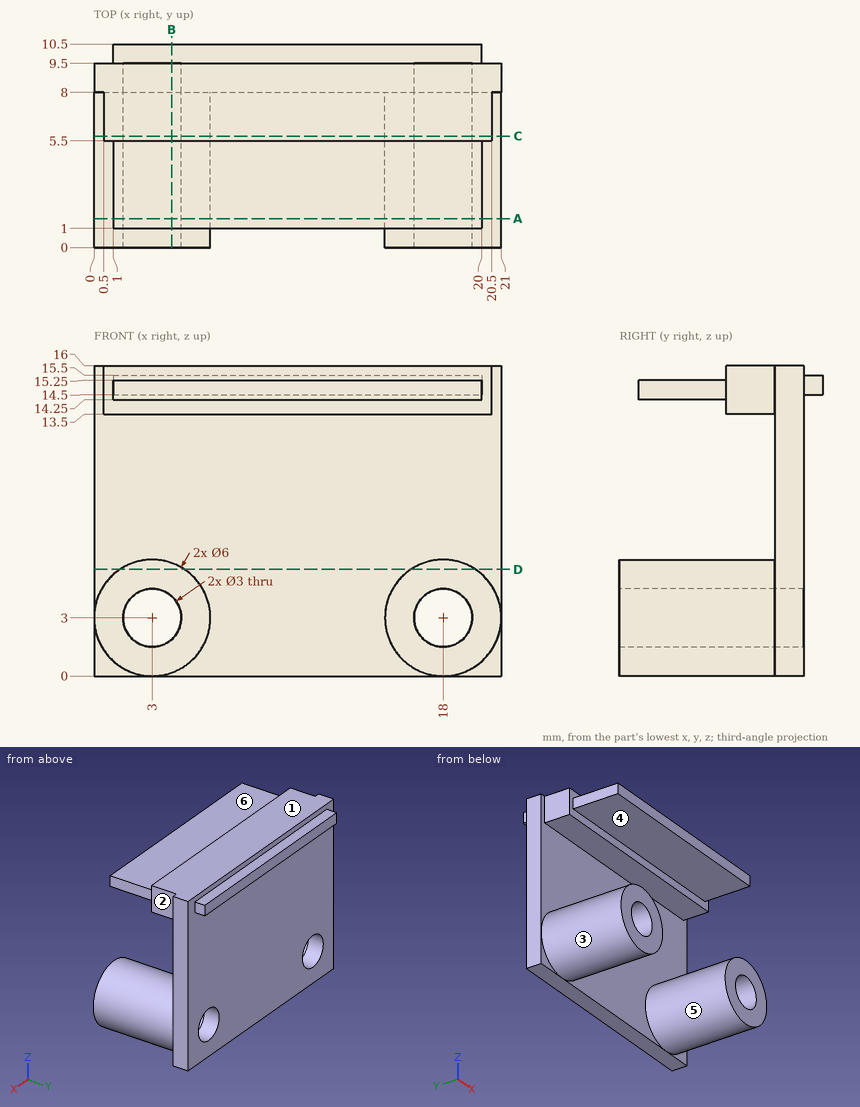
Here's the drawing with two shaded views (mm, measured from the low corner). I have some questions. A direction names the side the tool comes from. Coordinates: 2 decimals unless noted, no trailing zeros. Order: outer loops, then holes, each group sorted by start corner. A loop starts at its lowest first (then second) coordinate and runs counter-clockwise, first axis right, second up. Notation, with made-up numbers: (-13.5, 28.5) - (7.5, 28.5) arc R35 ccw to (7.5, 63.5) - close; hole circle Ø1 at (-23, 71). An arc over 180 degrees is marked (long way). Answer in a Markdown table with one row per item. Add a question column.
(1) If we section it at A-A, the plane y = 1.5: Please give me the cut outline in (x, z).
(2) If we mould it in two halves opening along Z, with no side actions, what happens to the marked faces 1, 2 and 3? For each: released by +Z, released by -Z, zero draft, split by the parting line, or undercut.
(3) I need wall thicknesses on L1, parallel to Z at x = 18, y = 6.5; L2, parallel to X at y = 2, z = 3; L3, parallel to Z at x = 2.25, y = 4.25. Which ranges of each line are inside material? Lowest first, please.
(4) Will these pins go through, and if not, where does the flat tip stop? pin 1 (0.8 mm diameter, centred on y = 7.5, z = 14.5, fed in from -X); pin 2 (1 mm diameter, centred on x = 14.5, z = 8, fed in from +Y); pin 3 (0.5 mm diameter, centred on y = 4, z = 14.5, fed in from +X).
(5) If we section it at B-B, the plane x = 4: Please give me the cut outline in (y, z), then the cut area to 3 significant figures.
(6) If we section it at D-D, the plane z = 5.5: Please give me the cut outline in (x, y), then the cut area to 3 significant figures.
(7) If we section it at C-C, the plane y = 5.75: Please give me the cut outline in (x, z), then the cut area to 3 significant figures.
(8) On a 3-axis mill with a long thin cutter (end or side, diameter ignored), from which of +Z, -Z, +X, -X, +Y, -Y can I reach the whole of each face in a straight line? I mean the marked faces 4, 5 and 6. Say none if no direction works.
Results are:
| question | item | result |
|---|---|---|
| 1 | outline | circle Ø6 at (3, 3); (1, 14.25) - (20, 14.25) - (20, 15.25) - (1, 15.25) - close; circle Ø6 at (18, 3); hole circle Ø3 at (3, 3); hole circle Ø3 at (18, 3) |
| 2 | face 1 | released by +Z |
| 2 | face 2 | zero draft |
| 2 | face 3 | undercut |
| 3 | L1 | z = 0 to 1.5, 4.5 to 6, 13.5 to 16 |
| 3 | L2 | x = 0 to 1.5, 4.5 to 6, 15 to 16.5, 19.5 to 21 |
| 3 | L3 | z = 0.1 to 1.7, 4.3 to 5.9, 14.25 to 15.25 |
| 4 | pin 1 | stops at x = 0.5 |
| 4 | pin 2 | stops at y = 9.5 |
| 4 | pin 3 | stops at x = 20 |
| 5 | outline | (0, 0.17) - (8, 0.17) - (8, 0) - (9.5, 0) - (9.5, 1.88) - (0, 1.88) - close; (0, 4.12) - (9.5, 4.12) - (9.5, 14.5) - (10.5, 14.5) - (10.5, 15.5) - (9.5, 15.5) - (9.5, 16) - (5.5, 16) - (5.5, 15.25) - (1, 15.25) - (1, 14.25) - (5.5, 14.25) - (5.5, 13.5) - (8, 13.5) - (8, 5.83) - (0, 5.83) - close |
| 5 | area | 59.8 mm2 |
| 6 | outline | (0, 8) - (1.34, 8) - (1.34, 0) - (4.66, 0) - (4.66, 8) - (16.34, 8) - (16.34, 0) - (19.66, 0) - (19.66, 8) - (21, 8) - (21, 9.5) - (0, 9.5) - close |
| 6 | area | 84.6 mm2 |
| 7 | outline | circle Ø6 at (3, 3); (0.5, 13.5) - (20.5, 13.5) - (20.5, 16) - (0.5, 16) - close; circle Ø6 at (18, 3); hole circle Ø3 at (3, 3); hole circle Ø3 at (18, 3) |
| 7 | area | 92.4 mm2 |
| 8 | face 4 | +X, -X, -Y |
| 8 | face 5 | -Y |
| 8 | face 6 | +Z, +X, -X, -Y |
